Read the model definition and answer for the solid it produces. Units are mm, in the model's axes. Face numbers are marked on the shaded views. A direction names the side the tool comes from. Give positions to 0.01 mm unless a question says otherwise; leave off trailing zeros. Write each loop counter-clockwise with the first axis right and the second up, starting at its lowest first coordinate (ties: lowest second). Pieces come first, ordered by that corner, then holes. Notation, with made-up numbers: M 6.25,46 L 21.25,46 A8 cw 21.25,58 Z; hole C 26,47 d9. An arc over 180 degrees is marked long. Put each result on its own line as item: value.
from build123d import *

# Parameters (mm, degrees)
F3_DEPTH = 152.401
F5_DEPTH = 152.401
F6_R     = 9.525


with BuildPart() as f1:
    # F0 (on Top) → F1 (revolve)
    with BuildSketch(Plane.XY):
        Polygon((-127, 19.05), (0, 19.05), (127, 19.05), (127, 38.1), (25.4, 38.1), (25.4, 177.8), (93.647316, 193.121127), (102.644078, 209.55), (121.419929, 209.55), (121.419929, 222.25), (114.3, 222.25), (114.3, 215.9), (95.063061, 215.9), (82.503349, 204.779378), (0, 184.872866), (-82.503349, 204.779378), (-95.063061, 215.9), (-114.3, 215.9), (-114.3, 222.25), (-121.419929, 222.25), (-121.419929, 209.55), (-102.644078, 209.55), (-93.647316, 193.121127), (-25.4, 177.8), (-25.4, 38.1), (-127, 38.1), align=None)
    revolve(axis=Axis((63.5, 0, 0), (1, 0, 0)))

    # F2 (on face) → F3 (cut, through all)
    with BuildSketch(Plane.YZ.offset(25.4)):
        with BuildLine():
            ThreePointArc((66.762265, 133.715989), (69.734989, 150.63986), (57.873824, 163.072367))
            ThreePointArc((57.873824, 163.072367), (0, 173.0375), (-57.873824, 163.072367))
            ThreePointArc((-57.873824, 163.072367), (-69.734989, 150.63986), (-66.762265, 133.715989))
            Line((-66.762265, 133.715989), (-15.259872, 64.796543))
            ThreePointArc((-15.259872, 64.796543), (0, 57.15), (15.259872, 64.796543))
            Line((15.259872, 64.796543), (66.762265, 133.715989))
        make_face()
        with BuildLine():
            ThreePointArc((-172.975032, -4.649144), (-164.816317, -19.771639), (-147.802138, -22.174174))
            Line((-147.802138, -22.174174), (-66.340734, 5.510233))
            ThreePointArc((-66.340734, 5.510233), (-54.35288, 17.660321), (-56.909615, 34.536233))
            Line((-56.909615, 34.536233), (-106.540789, 104.8152))
            ThreePointArc((-106.540789, 104.8152), (-121.717724, 112.872192), (-137.207042, 105.43341))
            ThreePointArc((-137.207042, 105.43341), (-164.568442, 53.471528), (-172.975032, -4.649144))
        make_face()
        with BuildLine():
            ThreePointArc((-49.030625, -165.945696), (-32.127097, -162.859405), (-24.584479, -147.420383))
            Line((-24.584479, -147.420383), (-25.740957, -61.391032))
            ThreePointArc((-25.740957, -61.391032), (-33.591927, -46.235321), (-50.431948, -43.451977))
            Line((-50.431948, -43.451977), (-132.608094, -68.936633))
            ThreePointArc((-132.608094, -68.936633), (-144.960679, -80.881009), (-142.672439, -97.910936))
            ThreePointArc((-142.672439, -97.910936), (-101.708891, -139.990278), (-49.030625, -165.945696))
        make_face()
        with BuildLine():
            ThreePointArc((142.672439, -97.910936), (144.960679, -80.881009), (132.608094, -68.936633))
            Line((132.608094, -68.936633), (50.431948, -43.451977))
            ThreePointArc((50.431948, -43.451977), (33.591927, -46.235321), (25.740957, -61.391032))
            Line((25.740957, -61.391032), (24.584479, -147.420383))
            ThreePointArc((24.584479, -147.420383), (32.127097, -162.859405), (49.030625, -165.945696))
            ThreePointArc((49.030625, -165.945696), (101.708891, -139.990278), (142.672439, -97.910936))
        make_face()
        with BuildLine():
            ThreePointArc((137.207042, 105.43341), (121.717724, 112.872192), (106.540789, 104.8152))
            Line((106.540789, 104.8152), (56.909615, 34.536233))
            ThreePointArc((56.909615, 34.536233), (53.63544, 26.400646), (54.35288, 17.660321))
            ThreePointArc((54.35288, 17.660321), (58.909893, 10.167549), (66.340734, 5.510233))
            Line((66.340734, 5.510233), (147.802138, -22.174174))
            ThreePointArc((147.802138, -22.174174), (164.816317, -19.771639), (172.975032, -4.649144))
            ThreePointArc((172.975032, -4.649144), (164.568442, 53.471528), (137.207042, 105.43341))
        make_face()
    extrude(amount=-F3_DEPTH, mode=Mode.SUBTRACT)

    # F4 (on face) → F5 (cut, through all)
    with BuildSketch(Plane.YZ.offset(25.4)):
        with BuildLine():
            Line((76.935513, 126.113685), (25.433119, 57.194239))
            ThreePointArc((25.433119, 57.194239), (28.214702, 38.834206), (46.535688, 41.862326))
            Line((46.535688, 41.862326), (96.166861, 112.141293))
            ThreePointArc((96.166861, 112.141293), (93.4441, 128.61477), (76.935513, 126.113685))
        make_face()
        with BuildLine():
            Line((-25.433119, 57.194239), (-76.935513, 126.113685))
            ThreePointArc((-76.935513, 126.113685), (-93.4441, 128.61477), (-96.166861, 112.141293))
            Line((-96.166861, 112.141293), (-46.535688, 41.862326))
            ThreePointArc((-46.535688, 41.862326), (-28.214702, 38.834206), (-25.433119, 57.194239))
        make_face()
        with BuildLine():
            Line((-62.25422, -6.514342), (-143.715623, -34.198749))
            ThreePointArc((-143.715623, -34.198749), (-151.19573, -49.126471), (-136.369902, -56.806555))
            Line((-136.369902, -56.806555), (-54.193756, -31.321899))
            ThreePointArc((-54.193756, -31.321899), (-45.652347, -14.833347), (-62.25422, -6.514342))
        make_face()
        with BuildLine():
            Line((-13.042105, -61.220324), (-11.885627, -147.249674))
            ThreePointArc((-11.885627, -147.249674), (0, -158.976599), (11.885627, -147.249674))
            Line((11.885627, -147.249674), (13.042105, -61.220324))
            ThreePointArc((13.042105, -61.220324), (0, -48.001718), (-13.042105, -61.220324))
        make_face()
        with BuildLine():
            Line((54.193756, -31.321899), (136.369902, -56.806555))
            ThreePointArc((136.369902, -56.806555), (151.19573, -49.126471), (143.715623, -34.198749))
            Line((143.715623, -34.198749), (62.25422, -6.514342))
            ThreePointArc((62.25422, -6.514342), (45.652347, -14.833347), (54.193756, -31.321899))
        make_face()
    extrude(amount=-F5_DEPTH, mode=Mode.SUBTRACT)

    # F6
    f6_edges = [f1.edges().sort_by_distance(p)[0] for p in [
        (25.4, -38.1, 0),
        (-25.4, -38.1, 0),
    ]]
    fillet(f6_edges, radius=F6_R)


solid = f1.part
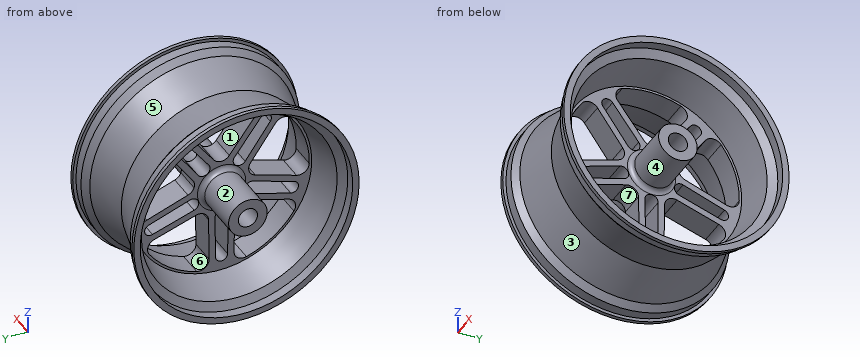
(1) Straight lines are drawn through the part: line 1 along Z through (x, y) = (-106, 0); line 2 along Z through (x, y) = (116, 0); line 3 along Y through (x, z) = (8.5, -94). For each, find the intervals that lie inside material, in ascending order. Write a range as from..to.
Result:
line 1: z = -215.9..-209.55, -38.1..-19.05, 19.05..38.1, 209.55..215.9
line 2: z = -222.25..-209.55, -38.1..-19.05, 19.05..38.1, 209.55..222.25
line 3: y = -161.57..-144.73, -25.3..-12.6, 12.6..25.3, 144.73..161.57
(2) Section B-B on z = 78 is taken. Give the number of separate pieces and of enclosed holes in the cut face, and give its area (3 significant figures).
Result:
separate pieces: 6
enclosed holes: 0
area: 10,400 mm²
(3) Given pin 1 Ø6 at (x, y) = (-17.5, -67) entering from +Z; pin 2 Ø23 at (y, z) = (0, 0) entering from +X; pin 3 Ø3 at (x, z) = (57, 132) entering from +Y; pin 4 Ø2 at (x, y) = (-10, 121) entering from -Z, each flat-ended and moving along its own axis, determine where each tip first touches the part or whether it passes through.
Result:
pin 1: stops at z = 178.18
pin 2: passes through
pin 3: stops at y = 149.83
pin 4: stops at z = -143.85
(4) Which of the six approach directions +Z, -Z, +X, -X, +Y, -Y give full straight-line access (tool end or side, diameter ignored) to the marked faces 1, 2, 3 and 4?
Result:
face 1: +X, -X
face 2: -X
face 3: none
face 4: +X
(5) Section A-A on x = -41 is taken. Determine the outline of the cut face in (y, z), and give its area (3 significant figures).
Result:
outline: C 0,0 d389.53; C 0,0 d76.2; hole C 0,0 d362.6; hole C 0,0 d38.1
area: 19,300 mm²
(6) For a pull along Z with two mould halves and no side action, classify the marked faces 5, 6 and 7 as +Z half, -Z half, draft (parallel to the pull), parting line (faces both ways), or undercut.
Result:
face 5: parting line
face 6: undercut
face 7: undercut
